Geometry: see drawing. Coordinates: mm, zero at the bounding-box minimum. A direction names the side the tool comes from. Round coordinates to 2 decimals unless told otherwise and drop trailing zeros. Order: outer loops, then holes, each group sorted by start corner. A loop starts at its lowest first (then second) coordinate and runs counter-clockwise, first axis right, second up. Notation, with made-up numbers: (-7, 23) -> (32, 23) arc R20 cw to (32, 33) -> close; hole circle Ø1 at (-7.5, 19). An arc over 180 degrees is marked (long way). Write item = value, one per line. Start each with the question number.
(1) Cut plane B-B on z = 20.9. Return the cut outline in (x, y).
(2) Contact query for a flat-ended pin moving along its axis: pin 1 Ø1.8 at (x, y) = (31, 3) entering from -Z. Output: stop coordinate, or through.
(3) Draft query along X for the marked faces 3, 4 and 5. Return one class per face: released by +X, released by -X, zero draft, split by the parting line, or undercut.
(4) Cut plane A-A on x = 17. Return the cut outline in (y, z), then the cut area to 3 significant figures.
(5) Reachability of the marked faces 1 and 2 from +Z, -Z, +X, -X, +Y, -Y: full face, straight path, thin tool, end or side. Return the list, or none.
(6) Cut plane C-C on y = 17.25. Return the cut outline in (x, z), then the cut area to 3 significant figures.
(7) Cut plane D-D on y = 14. Return the cut outline in (x, z).
(8) Ray query, line 1 (Y direction, x = 3, z = 19); line 2 (X direction, y = 7.5, z = 9.75); line 3 (X direction, y = 2.95, z = 9). Return the intervals inside material, ascending.
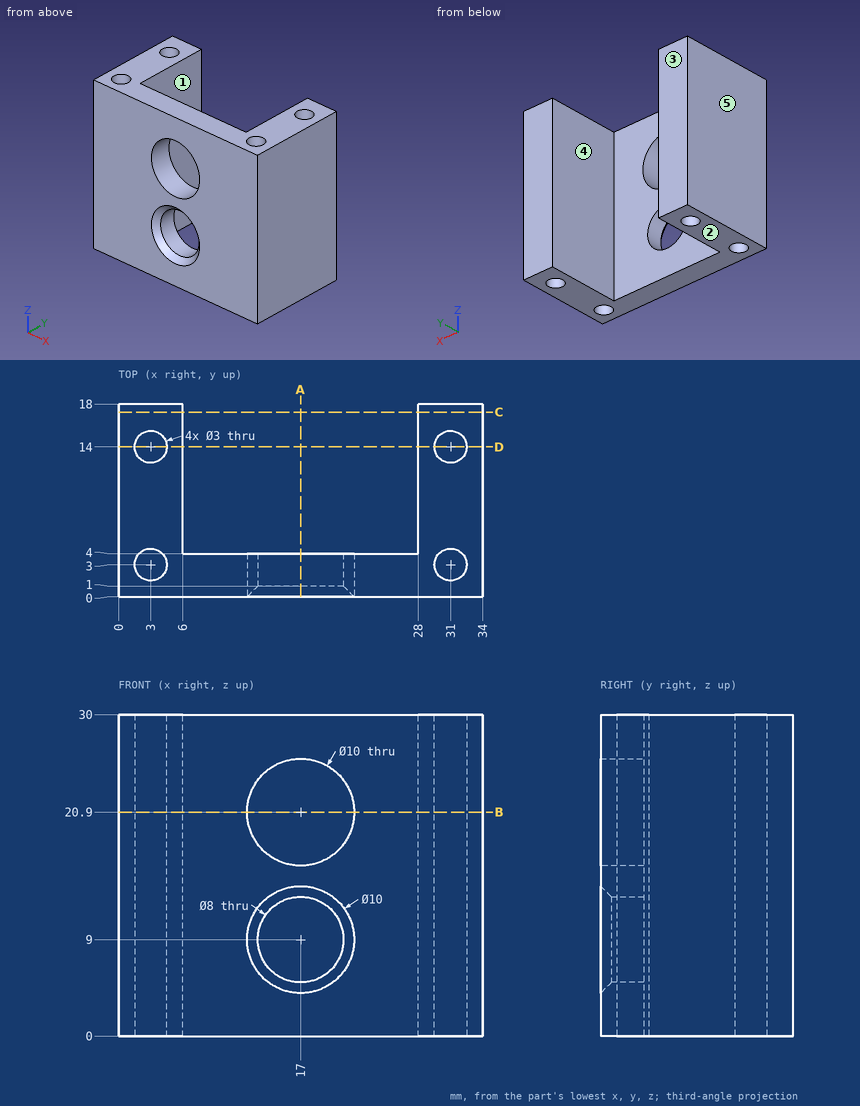
Evaluation:
q1.outline = (0, 0) -> (12, 0) -> (12, 4) -> (6, 4) -> (6, 18) -> (0, 18) -> close; (22, 0) -> (34, 0) -> (34, 18) -> (28, 18) -> (28, 4) -> (22, 4) -> close; hole circle Ø3 at (3, 3); hole circle Ø3 at (3, 14); hole circle Ø3 at (31, 3); hole circle Ø3 at (31, 14)
q2.pin_1 = through
q3.face_3 = zero draft
q3.face_4 = undercut
q3.face_5 = released by -X
q4.outline = (0, 0) -> (4, 0) -> (4, 5) -> (1, 5) -> (0, 4) -> close; (0, 14) -> (1, 13) -> (4, 13) -> (4, 15.9) -> (0, 15.9) -> close; (0, 25.9) -> (4, 25.9) -> (4, 30) -> (0, 30) -> close
q4.area = 47.0 mm^2
q5.face_1 = +Z, -Z, +Y
q5.face_2 = -Z, +X, -X, +Y, -Y
q6.outline = (0, 0) -> (6, 0) -> (6, 30) -> (0, 30) -> close; (28, 0) -> (34, 0) -> (34, 30) -> (28, 30) -> close
q6.area = 360 mm^2
q7.outline = (0, 0) -> (1.5, 0) -> (1.5, 30) -> (0, 30) -> close; (4.5, 0) -> (6, 0) -> (6, 30) -> (4.5, 30) -> close; (28, 0) -> (29.5, 0) -> (29.5, 30) -> (28, 30) -> close; (32.5, 0) -> (34, 0) -> (34, 30) -> (32.5, 30) -> close
q8.line_1 = 0 to 1.5, 4.5 to 12.5, 15.5 to 18
q8.line_2 = 0 to 6, 28 to 34
q8.line_3 = 0 to 1.5, 4.5 to 13, 21 to 29.5, 32.5 to 34
